Could you check a few things on this model? Use its own coordinates, in mm. A direction names the side the tool comes from. Give positions to 0.01 mm unless a question says otherwise; leave off trailing zeros. Loops run counter-clockwise (first coordinate to the right, second up) from the corner with the lowest first, then second, coordinate; pieces in that order, holes last. Notation, with made-up numbers: M 72.5,87.25 L 122.5,87.25 A7 cw 122.5,92.25 Z; hole C 30,-9 d2. An arc over 180 degrees is marked long. Answer in a Markdown table with one row per item. Add a question column.
1. I need wall thicknesses on line 1 along Y through (x, z) = (6.4, 0); line 2 along Z through (x, y) = (3.25, 0); line 3 along Y through (x, z) = (5.25, -160). Which ranges of each line are inside material? Lowest first, please. Write a range as from..to.
2. I'm going to push flat-ended pins straight in: pin 1 Ø3 at (y, z) = (-8.5, 0) entering from +X; pin 2 Ø1.5 at (x, y) = (6.5, -4.5) entering from -Z; pin 3 Ø1.8 at (x, z) = (4.5, -106) entering from +Y; pin 4 Ø3 at (x, z) = (1.5, -69) entering from -Y. Where does each tip first touch, or does it pass through?
3. If we section it at A-A on z = -8.5: List the corners of the cut face in (x, y) for me.
4. If we section it at B-B on z = -140.5: List the corners of the cut face in (x, y) for me.
5. Which directions (+Z, -Z, +X, -X, +Y, -Y) give clear straight access to the entire face, cutting with the end or side of a thin tool? Please do faces 1 (the cylindrical face through (6.479, -0.423, 5.278)), 2 (the cylindrical face through (2.46, 0.37, -10.16)), 3 (the flat face through (4, -10, -84)), 4 (the flat face through (8, 0, -78)), 5 (the flat face through (4, 10, -82)).
Autodesk Inventor part; units mm, degrees
ref_plane "YZ Plane" through (0, 0, 0) normal (1, 0, 0) x (0, 1, 0)
ref_plane "XZ Plane" through (0, 0, 0) normal (0, 1, 0) x (-1, 0, 0)
ref_plane "XY Plane" through (0, 0, 0) normal (0, 0, 1) x (1, 0, 0)
sketch "スケッチ1" plane through (0, 0, 0) normal (1, 0, 0) x (0, 1, 0)
  circle A0 centre (0, 0) radius 12
  line L0 (0, 0) -> (10, 0)
  line L1 (10, 0) -> (10, -170)
  line L2 (10, -170) -> (0, -170)
  line L3 (0, -170) -> (0, 0)
  point P0 (10, -6.6332)
  point P1 (0, -12)
  dimension "d0" = 24
  dimension "d1" = 170
  dimension "d2" = 10
extrude "押し出し1" add sketch "スケッチ1" along normal blind 8 contours A0 L1 L0 L3 | L3 L0 L1 A0
sketch "スケッチ2" plane through (8, 0, 0) normal (1, 0, 0) x (0, 0, -1)
  circle A0 centre (0, 0) radius 8.5
  point P0 (0, 8.5)
  dimension "d7" = 17
hole "穴1" at (8, 8.5, 0) direction (-1, 0, 0) diameter 3.4 end through all counterbore diameter 6.5 counterbore depth 3
pattern_circular "円形状パターン1" count 4 over 360 about axis through (0, 0, 0) along (1, 0, 0) of "穴1"
extrude "押し出し2" add sketch "スケッチ1" along normal blind 8 contours A0 L1 L2 L3
mirror "ミラー1" about plane through (0, 0, 0) normal (0, 1, 0) of "押し出し2"
sketch "スケッチ4" plane through (8, 0, 0) normal (1, 0, 0) x (0, 0, -1)
  line L0 (170, 10) -> (170, -10)
  point P0 (0, 0)
  point P1 (160, 0)
  dimension "d23" = 10
hole "穴2" at (8, 0, -160) direction (-1, 0, 0) diameter 12.3 end through all
fillet "フィレット1" radius 10 2 edges at (4, 10, -170) (4, -10, -170)
fillet "フィレット2" radius 1 6 edges at (8, -10, -83.3169) (8, 10, -83.3169) (8, 0, 12) (0, -10, -83.3169) (0, 10, -83.3169) (0, 0, 12)
sketch "スケッチ3" plane through (8, 0, 0) normal (1, 0, 0) x (0, 0, -1)
  point P0 (0, 0)
properties part number "base5" material "ABS プラスチック"
Results:
| question | item | result |
|---|---|---|
| 1 | line 1 | -12..-11.75, -5.25..5.25, 11.75..12 |
| 1 | line 2 | -170..-166.15, -153.85..-10.2, -6.8..6.8, 10.2..12 |
| 1 | line 3 | -10..-6.15, 6.15..10 |
| 2 | pin 1 | through |
| 2 | pin 2 | z = -169.27 |
| 2 | pin 3 | y = 10 |
| 2 | pin 4 | y = -10 |
| 3 | outline | M 0,-9 A1 ccw 1,-10 L 7,-10 A1 ccw 8,-9 L 8,-3.25 L 5,-3.25 L 5,-1.7 L 0,-1.7 Z; M 0,1.7 L 5,1.7 L 5,3.25 L 8,3.25 L 8,9 A1 ccw 7,10 L 1,10 A1 ccw 0,9 Z |
| 4 | outline | M 0,-9 A1 ccw 1,-10 L 7,-10 A1 ccw 8,-9 L 8,9 A1 ccw 7,10 L 1,10 A1 ccw 0,9 Z |
| 5 | face 1 | +X |
| 5 | face 2 | +X, -X |
| 5 | face 3 | -Z, +X, -X, -Y |
| 5 | face 4 | +Z, -Z, +X, +Y, -Y |
| 5 | face 5 | -Z, +X, -X, +Y |
